from build123d import *

# Parameters (mm, degrees)
SKETCH_1_W          = 20
SKETCH_1_H          = 17.5
EXTRUDE_1_DEPTH     = 1000
CUT_EXTRUDE_1_DEPTH = 1001.088277354
SKETCH_3_R          = 3
CUT_EXTRUDE_2_DEPTH = 1001.203104374
SKETCH_4_R          = 4.75
CUT_EXTRUDE_3_DEPTH = 10


with BuildPart() as part:
    # 草图1 → 凸台-拉伸1 (new body)
    with BuildSketch(Plane(origin=(0, 0, 0), x_dir=(1, 0, 0), z_dir=(0, 1, 0))):
        Rectangle(SKETCH_1_W, SKETCH_1_H)
    extrude(amount=EXTRUDE_1_DEPTH)

    # 草图2 → 切除-拉伸1 (cut, through all)
    with BuildSketch(Plane.XZ):
        Polygon((-8, 8.75), (-10, 6.75), (-10, 8.75), align=None)
        Polygon((10, 6.75), (8, 8.75), (10, 8.75), align=None)
        Polygon((10, 2.25), (7, -0.75), (7, -4.75), (10, -7.75), align=None)
        Polygon((-7, -4.75), (-10, -7.75), (-10, 2.25), (-7, -0.75), align=None)
    extrude(amount=-CUT_EXTRUDE_1_DEPTH, mode=Mode.SUBTRACT)

    # 草图3 → 切除-拉伸2 (cut, through all)
    with BuildSketch(Plane.XY.offset(8.75)):
        with Locations((0, 980)):
            Circle(SKETCH_3_R)
        with Locations((0, 920)):
            Circle(SKETCH_3_R)
        with Locations((0, 860)):
            Circle(SKETCH_3_R)
        with Locations((0, 800)):
            Circle(SKETCH_3_R)
        with Locations((0, 740)):
            Circle(SKETCH_3_R)
        with Locations((0, 680)):
            Circle(SKETCH_3_R)
        with Locations((0, 620)):
            Circle(SKETCH_3_R)
        with Locations((0, 560)):
            Circle(SKETCH_3_R)
        with Locations((0, 500)):
            Circle(SKETCH_3_R)
        with Locations((0, 440)):
            Circle(SKETCH_3_R)
        with Locations((0, 380)):
            Circle(SKETCH_3_R)
        with Locations((0, 320)):
            Circle(SKETCH_3_R)
        with Locations((0, 260)):
            Circle(SKETCH_3_R)
        with Locations((0, 200)):
            Circle(SKETCH_3_R)
        with Locations((0, 140)):
            Circle(SKETCH_3_R)
        with Locations((0, 80)):
            Circle(SKETCH_3_R)
        with Locations((0, 20)):
            Circle(SKETCH_3_R)
    extrude(amount=-CUT_EXTRUDE_2_DEPTH, mode=Mode.SUBTRACT)

    # 草图4 → 切除-拉伸3 (cut)
    with BuildSketch(Plane.XY.offset(8.75)):
        with Locations((0, 980)):
            Circle(SKETCH_4_R)
        with Locations((0, 920)):
            Circle(SKETCH_4_R)
        with Locations((0, 860)):
            Circle(SKETCH_4_R)
        with Locations((0, 800)):
            Circle(SKETCH_4_R)
        with Locations((0, 740)):
            Circle(SKETCH_4_R)
        with Locations((0, 680)):
            Circle(SKETCH_4_R)
        with Locations((0, 620)):
            Circle(SKETCH_4_R)
        with Locations((0, 560)):
            Circle(SKETCH_4_R)
        with Locations((0, 500)):
            Circle(SKETCH_4_R)
        with Locations((0, 440)):
            Circle(SKETCH_4_R)
        with Locations((0, 380)):
            Circle(SKETCH_4_R)
        with Locations((0, 320)):
            Circle(SKETCH_4_R)
        with Locations((0, 260)):
            Circle(SKETCH_4_R)
        with Locations((0, 200)):
            Circle(SKETCH_4_R)
        with Locations((0, 140)):
            Circle(SKETCH_4_R)
        with Locations((0, 80)):
            Circle(SKETCH_4_R)
        with Locations((0, 20)):
            Circle(SKETCH_4_R)
    extrude(amount=-CUT_EXTRUDE_3_DEPTH, mode=Mode.SUBTRACT)


solid = part.part
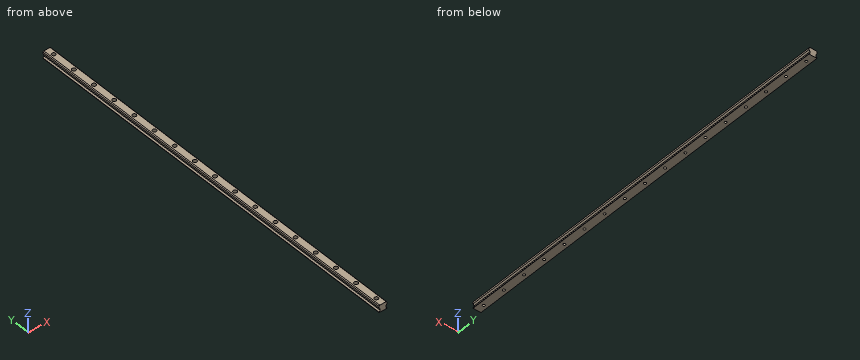
Build history of the part. All positions in model axes, mm. Give positions to 0.01 mm unless a question says otherwise; leave off trailing zeros. Order: outer loops, then holes, each group sorted by start corner. A loop starts at its lowest first (then second) coordinate and runs counter-clockwise, first axis right, second up. Notation, with made-up numbers: M 8,48.25 L 55,48.25 A23 cw 55,60.25 Z; hole C -1.5,20 d11. An arc over 180 degrees is marked long. Put each result on its own line as item: value.
Item 1: Probe line 1 (X direction, y = 860, z = 3.5); line 2 (X direction, y = 740, z = -3); line 3 (Z direction, x = -8.75, y = 567.5). List the from-to ranges inside material, lowest first. Write a range as [from, to].
From the geometry:
line 1: x = [-10, -4.75], [4.75, 10]
line 2: x = [-7, -3], [3, 7]
line 3: z = [-8.75, -6.5], [1, 8]
Item 2: Slice it at B-B, the plane x = 0. Give the number of separate pieces and of enclosed holes in the cut face, plus the area to 3 significant figures.
From the geometry:
separate pieces: 18
enclosed holes: 0
area: 15,100 mm2
Item 3: Flat gauge pins, fed straight in: pin 1 Ø3.5 at (x, y) = (0, 740) entering from +Z; pin 2 Ø1.2 at (y, z) = (702.5, -2) entering from +X; pin 3 Ø5 at (x, y) = (-2, 560.5) entering from +Z; pin 4 Ø2 at (y, z) = (770, -5.5) entering from +X. Where does each tip first touch, or does it go through?
From the geometry:
pin 1: passes through
pin 2: stops at x = 7
pin 3: stops at z = -1.25
pin 4: stops at x = 8.75
Item 4: Slice it at A-A, the plane y = 828. Write the cut outline in (x, z).
From the geometry:
outline: M -10,-8.75 L 10,-8.75 L 10,-7.75 L 7,-4.75 L 7,-0.75 L 10,2.25 L 10,6.75 L 8,8.75 L -8,8.75 L -10,6.75 L -10,2.25 L -7,-0.75 L -7,-4.75 L -10,-7.75 Z
